```python
from build123d import *

# Parameters (mm, degrees)
CHAMFER2_SIZE      = 1
CUT_EXTRUDE1_START = -111
CUT_EXTRUDE1_DEPTH = 111
SKETCH3_W          = 6.659868337
SKETCH3_H          = 5.59204707
CUT_EXTRUDE2_DEPTH = 1
SKETCH4_W          = 5.737170607
SKETCH4_H          = 4.399946053
CUT_EXTRUDE3_DEPTH = 2
CUT_EXTRUDE4_DEPTH = 2
SKETCH6_W          = 0.57084709
SKETCH6_H          = 1.008895736
CUT_EXTRUDE5_DEPTH = 2


with BuildPart() as part:
    # Sketch1 → Revolve1 (revolve)
    with BuildSketch(Plane.XY, mode=Mode.PRIVATE) as revolve1_sk:
        Polygon((43.331874727, 0), (109.831874727, 0), (109.831874727, -21), (103.831874727, -21), (103.831874727, -22.25), (63.831874727, -22.25), (63.831874727, -21), (43.331874727, -21), align=None)
    revolve(revolve1_sk.sketch.rotate(Axis((169.06951142, 0, 0), (-1, 0, 0)), 180), axis=Axis((169.06951142, 0, 0), (-1, 0, 0)))

    # Chamfer2
    chamfer2_edges = [part.edges().sort_by_distance(p)[0] for p in [
        (109.831874727, -21, 0),
    ]]
    chamfer(chamfer2_edges, length=CHAMFER2_SIZE)

    # Sketch2 → Cut-Extrude1 (cut)
    with BuildSketch(Plane(origin=(103.831874727, 0, 0), x_dir=(0, 0, -1), z_dir=(1, 0, 0)).offset(CUT_EXTRUDE1_START)):
        with BuildLine():
            Line((-4.120122391, 21.865202754), (-3.888654841, 20.636820577))
            ThreePointArc((-3.888654841, 20.636820577), (0, 21), (3.888654841, 20.636820577))
            Line((3.888654841, 20.636820577), (4.120122391, 21.865202754))
            ThreePointArc((4.120122391, 21.865202754), (0, 22.25), (-4.120122391, 21.865202754))
        make_face()
        with BuildLine():
            ThreePointArc((3.888654841, -20.636820577), (0, -21), (-3.888654841, -20.636820577))
            Line((-3.888654841, -20.636820577), (-4.120122391, -21.865202754))
            ThreePointArc((-4.120122391, -21.865202754), (0, -22.25), (4.120122391, -21.865202754))
            Line((4.120122391, -21.865202754), (3.888654841, -20.636820577))
        make_face()
    extrude(amount=CUT_EXTRUDE1_DEPTH, mode=Mode.SUBTRACT)

    # Sketch3 → Cut-Extrude2 (cut)
    with BuildSketch(Plane(origin=(0, 21, 0), x_dir=(1, 0, 0), z_dir=(0, 1, 0))):
        with Locations((46.661808896, 0.080549256)):
            Rectangle(SKETCH3_W, SKETCH3_H)
    extrude(amount=-CUT_EXTRUDE2_DEPTH, mode=Mode.SUBTRACT)

    # Sketch4 → Cut-Extrude3 (cut)
    with BuildSketch(Plane(origin=(0, 20, 0), x_dir=(1, 0, 0), z_dir=(0, 1, 0))):
        with Locations((46.200460031, 0.055345837)):
            Rectangle(SKETCH4_W, SKETCH4_H)
    extrude(amount=-CUT_EXTRUDE3_DEPTH, mode=Mode.SUBTRACT)

    # Sketch5 → Cut-Extrude4 (cut)
    with BuildSketch(Plane.ZY.offset(-43.331874727)):
        with BuildLine():
            ThreePointArc((14.925071035, 13.313236068), (13.674240438, 14.595038488), (12.31375629, 15.759803489))
            ThreePointArc((12.31375629, 15.759803489), (7.517637174, 18.533351864), (2.144627189, 19.884681899))
            Line((2.144627189, 19.884681899), (2.144627189, 18))
            Line((2.144627189, 18), (-2.255318864, 18))
            Line((-2.255318864, 18), (-2.255318864, 19.872431578))
            ThreePointArc((-2.255318864, 19.872431578), (-5.211421697, 19.309093296), (-8.049539324, 18.308602259))
            ThreePointArc((-8.049539324, 18.308602259), (-9.655133779, 17.5150904), (-11.183303846, 16.581125266))
            ThreePointArc((-11.183303846, 16.581125266), (-18.10627914, 8.494860547), (-19.899959931, -1.997897586))
            ThreePointArc((-19.899959931, -1.997897586), (-19.641441279, -3.770117305), (-19.225418173, -5.512104503))
            ThreePointArc((-19.225418173, -5.512104503), (-13.674240438, -14.595038488), (-4.249312288, -19.543370873))
            ThreePointArc((-4.249312288, -19.543370873), (-2.483944519, -19.845151036), (-0.698658033, -19.987793199))
            ThreePointArc((-0.698658033, -19.987793199), (9.655133779, -17.5150904), (17.273740508, -10.080569868))
            ThreePointArc((17.273740508, -10.080569868), (18.10627914, -8.494860547), (18.793623762, -6.841031054))
            ThreePointArc((18.793623762, -6.841031054), (19.696097015, -3.473292728), (20, 0))
            ThreePointArc((20, 0), (18.688250596, 7.123853568), (14.925071035, 13.313236068))
        make_face()
        with BuildLine():
            Line((2.144627189, 18), (2.144627189, 19.884681899))
            ThreePointArc((2.144627189, 19.884681899), (-0.055683744, 19.999922483), (-2.255318864, 19.872431578))
            Line((-2.255318864, 19.872431578), (-2.255318864, 18))
            Line((-2.255318864, 18), (2.144627189, 18))
        make_face()
        with BuildLine():
            ThreePointArc((-11.183303846, 16.581125266), (-9.655133779, 17.5150904), (-8.049539324, 18.308602259))
            Line((-8.049539324, 18.308602259), (-8.45201629, 19.224032372))
            ThreePointArc((-8.45201629, 19.224032372), (-10.137890468, 18.39084492), (-11.742469038, 17.410181529))
            Line((-11.742469038, 17.410181529), (-11.183303846, 16.581125266))
        make_face()
        with BuildLine():
            Line((12.929444105, 16.547793664), (12.31375629, 15.759803489))
            ThreePointArc((12.31375629, 15.759803489), (13.674240438, 14.595038488), (14.925071035, 13.313236068))
            Line((14.925071035, 13.313236068), (15.671324586, 13.978897872))
            ThreePointArc((15.671324586, 13.978897872), (14.357952459, 15.324790412), (12.929444105, 16.547793664))
        make_face()
        with BuildLine():
            Line((19.733304951, -7.183082606), (18.793623762, -6.841031054))
            ThreePointArc((18.793623762, -6.841031054), (18.10627914, -8.494860547), (17.273740508, -10.080569868))
            Line((17.273740508, -10.080569868), (18.137427533, -10.584598362))
            ThreePointArc((18.137427533, -10.584598362), (19.011593097, -8.919603575), (19.733304951, -7.183082606))
        make_face()
        with BuildLine():
            Line((-0.733590935, -20.987182859), (-0.698658033, -19.987793199))
            ThreePointArc((-0.698658033, -19.987793199), (-2.483944519, -19.845151036), (-4.249312288, -19.543370873))
            Line((-4.249312288, -19.543370873), (-4.461777902, -20.520539417))
            ThreePointArc((-4.461777902, -20.520539417), (-2.608141745, -20.837408587), (-0.733590935, -20.987182859))
        make_face()
        with BuildLine():
            ThreePointArc((-19.225418173, -5.512104503), (-19.641441279, -3.770117305), (-19.899959931, -1.997897586))
            Line((-19.899959931, -1.997897586), (-20.894957927, -2.097792465))
            ThreePointArc((-20.894957927, -2.097792465), (-20.623513343, -3.95862317), (-20.186689082, -5.787709728))
            Line((-20.186689082, -5.787709728), (-19.225418173, -5.512104503))
        make_face()
    extrude(amount=-CUT_EXTRUDE4_DEPTH, mode=Mode.SUBTRACT)

    # Sketch6 → Cut-Extrude5 (cut)
    with BuildSketch(Plane.ZY.offset(-43.331874727)):
        with Locations((2.430050734, 20.319245355)):
            Rectangle(SKETCH6_W, SKETCH6_H)
        Polygon((-2.876572791, 20.802051076), (-2.876572791, 19.720628681), (-2.255318864, 19.720628681), (-2.255318864, 20.908214592), (-2.876572791, 20.908214592), align=None)
    extrude(amount=-CUT_EXTRUDE5_DEPTH, mode=Mode.SUBTRACT)


solid = part.part
```
Check sheet for the modelled part. Datum: model origin and axes. Units: mm. A direction names the side the tool comes from. Coordinates: 2 decimals unless noted, no trailing zeros. Order: outer loops, then holes, each group sorted by start corner. A loop starts at its lowest first (then second) coordinate and runs counter-clockwise, first axis right, second up. Notation, with made-up numbers: (12.25, -5) -> (47.25, -5) arc R13 ccw to (47.25, 14) -> close; hole circle Ø6 at (2.25, 78). An arc over 180 degrees is marked (long way). Write each question's results on one line, items separated by ' | '. Start each with the question number.
1) Depth check by flat-ended pin: pin 1 (8 mm diameter, centred on x = 52.5, z = 13.5, fed in from -Y); pin 2 (6 mm diameter, centred on x = 85, y = -15.5, fed in from -Z); pin 3 (20 mm diameter, centred on y = -1.5, z = 15.5, fed in from -X); pin 4 (5 mm diameter, centred on x = 48.5, z = -1, fed in from +Y). Enter the tip coordinate at first touch or a pass-through.
2) Set-up check for faces 4 (the face through (49.7, 20, -0.1)), 5 (the face through (103.832, 0.1, 21.2)), 6 (the face through (44.318, 18.395, 7.851)): record each of +Z, -Z, +X, -X, +Y, -Y from which the full face is reachable in a straight line by a thin tool's end or side.
3) Section check B-B (x = 62). Enter the section's corners in (y, z).
4) Section check A-A (x = 85). Enter the section's corners in (y, z).
5) Material ranges on line 1 along X through (y, z) = (-10.5, 6); line 2 along Z through (x, y) = (104.5, 0.5); line 3 along Z through (x, y) = (74.5, 9.5), recorded low to high.
6) Draft check along Z on faces 1 (the face through (49.069, 19, 0)), 2 (the face through (63.832, -0.1, -21.3)), 3 (the face through (83.552, -0.431, 22.246)). Enter one of: pulls with the +Z half, pulls with the -Z half, needs draft (parallel to the pull), parting line crosses it, or undercut.
Checked values:
1) pin 1: y = -18.73 | pin 2: z = -18.41 | pin 3: x = 43.33 | pin 4: y = 21
2) face 4: -X, +Y | face 5: +Z, +X | face 6: -X
3) outline: circle Ø42 at (0, 0)
4) outline: (-21.87, -4.12) arc R22.25 ccw to (21.87, -4.12) -> (20.64, -3.89) arc R21 ccw to (20.64, 3.89) -> (21.87, 4.12) arc R22.25 ccw to (-21.87, 4.12) -> (-20.64, 3.89) arc R21 ccw to (-20.64, -3.89) -> close
5) line 1: 45.33 to 109.83 | line 2: -20.99 to 20.99 | line 3: -20.12 to 20.12
6) face 1: undercut | face 2: needs draft | face 3: pulls with the +Z half
